from build123d import *

# Parameters (mm, degrees)
BOSS_EXTRUDE1_DEPTH       = 19
CUT_REVOLVE_THIN4_START   = 9.090052714
CUT_REVOLVE_THIN4_DEPTH   = 0.819894572
CUT_REVOLVE_THIN4_START_2 = 9.100052714
CUT_REVOLVE_THIN4_2_DEPTH = 0.799894572


with BuildPart() as part:
    # Sketch1 → Boss-Extrude1 (new body)
    with BuildSketch(Plane(origin=(0, 0, 0), x_dir=(1, 0, 0), z_dir=(0, 1, 0))):
        with BuildLine():
            Line((0, -10), (0, -11.5))
            ThreePointArc((0, -11.5), (8.131727984, -8.131727984), (11.5, 0))
            ThreePointArc((11.5, 0), (8.131727984, 8.131727984), (0, 11.5))
            Line((0, 11.5), (0, 10))
            ThreePointArc((0, 10), (7.071067812, 7.071067812), (10, 0))
            ThreePointArc((10, 0), (7.071067812, -7.071067812), (0, -10))
        make_face()
    extrude(amount=BOSS_EXTRUDE1_DEPTH)

    # Cut-Revolve-Thin4: read off the stored shape, not the designer's step
    # Cut-Revolve-Thin4 outline → Cut-Revolve-Thin4 (cut)
    with BuildSketch(Plane(origin=(0, 0, 0), x_dir=(1, 0, 0), z_dir=(0, 1, 0)).offset(CUT_REVOLVE_THIN4_START)):
        with BuildLine():
            ThreePointArc((0, -10.385), (10.385, 0), (0, 10.385))
            Line((0, 10.385), (0, 10))
            ThreePointArc((0, 10), (10, 0), (0, -10))
            Line((0, -10), (0, -10.385))
        make_face()
    extrude(amount=CUT_REVOLVE_THIN4_DEPTH, mode=Mode.SUBTRACT)


with BuildPart() as body_2:
    # Cut-Revolve-Thin4 2 outline → Cut-Revolve-Thin4 2 (new body)
    with BuildSketch(Plane(origin=(0, 0, 0), x_dir=(1, 0, 0), z_dir=(0, 1, 0)).offset(CUT_REVOLVE_THIN4_START_2)):
        with BuildLine():
            Line((0, 10.375), (0, 10))
            ThreePointArc((0, 10), (10, 0), (0, -10))
            Line((0, -10), (0, -10.375))
            ThreePointArc((0, -10.375), (10.375, 0), (0, 10.375))
        make_face()
    extrude(amount=CUT_REVOLVE_THIN4_2_DEPTH)


solid = part.part
For this review, take the finished solid that the model builds, in its own axes (mm). A direction names the side the tool comes from. Coordinates: 2 decimals unless noted, no trailing zeros. Order: outer loops, then holes, each group sorted by start corner. A loop starts at its lowest first (then second) coordinate and runs counter-clockwise, first axis right, second up. Notation, with made-up numbers: (59, 58) - (87, 58) arc R18 ccw to (87, 76) - close; hole circle Ø1 at (-36, 67). An arc over 180 degrees is marked (long way). Answer as CSV lines item,"result". Start each with the question number.
1) To check wall thickness, follow line 1 along Y through (x, z) = (6.75, 7.75); line 2 along Z through (x, y) = (3.25, 15.25); line 3 along Z through (x, y) = (0.5, 9.5). State the ranges of each line that lie inside material, in increasing order. Write a range as [from, to].
2) Add section C-C (z = 2). State the section outline as (x, y) points, then the cut area to 3 significant figures.
3) Add section D-D (x = 4.5). State the section outline as (y, z) points.
4) Add section A-A (x = 1.75). State the section outline as (y, z) points.
5) Insertion check: P1, Ø1.5, axis at x = 9.5, z = -1.5, coming from the +Y side; P2, Ø1, axis at x = 1.5, y = 11.5, coming from the -Z side; P3, Ø6, axis at y = 9, z = -9, coming from the +X side; P4, Ø1, axis at y = 8.5, z = 0, coming from the -X side. Each pin has a flat end and moves straight along its axis. Give the tip position at first contact, or say it passes through.
6) Add section B-B (y = 2.25). State the section outline as (x, z) points.
7) Machinability: for faces 1 (the flat face through (10.2, 9.91, -0.8)), 2 (the flat face through (0, 9, 11)), which of the approach directions +Z, -Z, +X, -X, +Y, -Y give a long, thin tool a straight path to every point of the face, cutting with its end or side? Answer none if there is none.
8) Draft analysis for pull direction Y (two halves, no side actions). For faces 3 (the cylindrical face through (10.382, 9.494, 0.228)), 4 (the flat face through (0, 9, -11)), 5 (the flat face through (10, 0, 2)), 6 (the flat face through (10, 19, 2)), state which applies: +Y half, -Y half, draft (parallel to the pull), parting line (faces both ways), or undercut.
Result:
1,line 1,"[0, 9.09], [9.91, 19]"
1,line 2,"[-11.03, -9.46], [9.46, 11.03]"
1,line 3,"[-11.49, -10.37], [10.37, 11.49]"
2,outline,"(9.8, 0) - (11.32, 0) - (11.32, 19) - (9.8, 19) - (9.8, 9.91) - (10.19, 9.91) - (10.19, 9.09) - (9.8, 9.09) - close"
2,area,"28.7 mm^2"
3,outline,"(0, -10.58) - (19, -10.58) - (19, -8.93) - (9.91, -8.93) - (9.91, -9.36) - (9.09, -9.36) - (9.09, -8.93) - (0, -8.93) - close; (0, 8.93) - (9.09, 8.93) - (9.09, 9.36) - (9.91, 9.36) - (9.91, 8.93) - (19, 8.93) - (19, 10.58) - (0, 10.58) - close"
4,outline,"(0, -11.37) - (19, -11.37) - (19, -9.85) - (9.91, -9.85) - (9.91, -10.24) - (9.09, -10.24) - (9.09, -9.85) - (0, -9.85) - close; (0, 9.85) - (9.09, 9.85) - (9.09, 10.24) - (9.91, 10.24) - (9.91, 9.85) - (19, 9.85) - (19, 11.37) - (0, 11.37) - close"
5,P1,"y = 19"
5,P2,"z = -11.46"
5,P3,"x = 9.81"
5,P4,"x = 9.99"
6,outline,"(0, -11.5) arc R11.5 ccw to (0, 11.5) - (0, 10) arc R10 cw to (0, -10) - close"
7,face 1,"-X"
7,face 2,"+Z, -Z, -X, +Y, -Y"
8,face 3,"undercut"
8,face 4,"draft"
8,face 5,"-Y half"
8,face 6,"+Y half"
